Geometry check sheet. Reference: drawing and pictorial views, mm from the part's lowest x, y, z. A direction names the side the tool comes from. Coordinates: 2 decimals unless noted, no trailing zeros. Order: outer loops, then holes, each group sorted by start corner. A loop starts at its lowest first (then second) coordinate and runs counter-clockwise, first axis right, second up. Notation, with made-up numbers: M -24,41.5 L 2,41.5 A26 cw 2,63.5 Z; hole C -10,-28 d1. An arc over 180 degrees is marked long. Return JSON: item names as keys, results as strings.
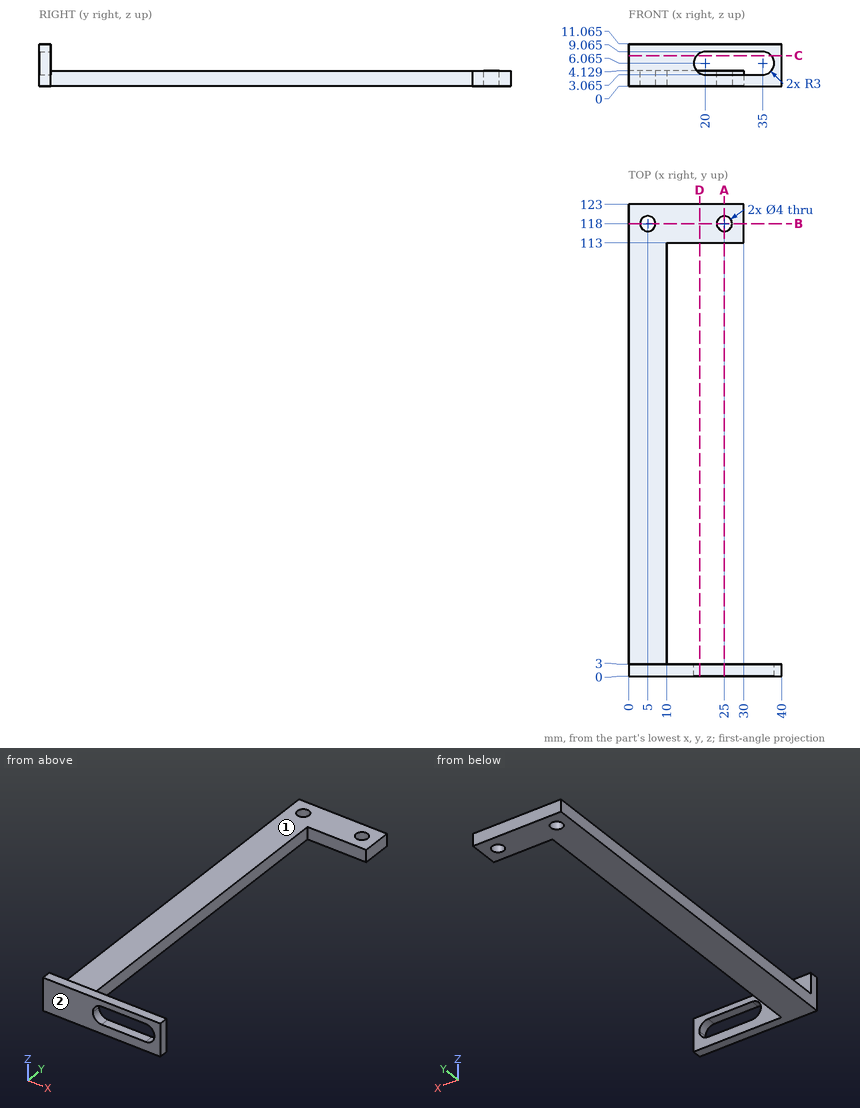
Q1. Tool access check on the marked faces 1 and 2. Record the directions out of +Z, -Z, +X, -X, +Y, -Y that give a thin tool (end or side, any length) a straight path to the whole face; none if there is none.
Values:
{"face 1": "+Z, +X, -X, +Y", "face 2": "+Z, -Z, +X, -X, -Y"}
Q2. Cross-section at B-B, the plane y = 118. Record the boundary of the cut face in (x, z).
Values:
{"outline": "M 0,0 L 3,0 L 3,4.13 L 0,4.13 Z; M 7,0 L 23,0 L 23,4.13 L 7,4.13 Z; M 27,0 L 30,0 L 30,4.13 L 27,4.13 Z"}
Q3. Cross-section at A-A, the plane x = 25. Record the boundary of the cut face in (y, z) (1 decimal).
Values:
{"outline": "M 0,0 L 3,0 L 3,3.1 L 0,3.1 Z; M 0,9.1 L 3,9.1 L 3,11.1 L 0,11.1 Z; M 113,0 L 116,0 L 116,4.1 L 113,4.1 Z; M 120,0 L 123,0 L 123,4.1 L 120,4.1 Z"}
Q4. Material ranges on line 1 along Y through (x, z) = (13.5, 1); line 2 along Y through (x, z) = (5, 2.35); line 3 along Y through (x, z) = (8, 6), recorded low to high.
Values:
{"line 1": "0 to 3, 113 to 123", "line 2": "0 to 116, 120 to 123", "line 3": "0 to 3"}
Q5. Cross-section at C-C, the plane z = 8. Record the boundary of the cut face in (x, y).
Values:
{"outline": "M 0,0 L 17.71,0 L 17.71,3 L 0,3 Z; M 37.29,0 L 40,0 L 40,3 L 37.29,3 Z"}
Q6. Go/stop test with flat-tipped pins: pin 1 (10 mm diameter, centred on x = 8.5, y = 29.5, fed in from +Z); pin 2 (2 mm diameter, centred on y = 63.5, z = 2, fed in from +X); pin 3 (3.5 mm diameter, centred on y = 120, z = 2.5, fed in from +X); pin 4 (3 mm diameter, centred on x = 25, y = 118, fed in from -Z). Record where each tip stops, or that it passes through.
Values:
{"pin 1": "z = 4.13", "pin 2": "x = 10", "pin 3": "x = 30", "pin 4": "through"}
Q7. Cross-section at D-D, the plane x = 18.5. Record the boundary of the cut face in (y, z) (1 decimal), and give its area (3 significant figures).
Values:
{"outline": "M 0,0 L 3,0 L 3,3.5 L 0,3.5 Z; M 0,8.7 L 3,8.7 L 3,11.1 L 0,11.1 Z; M 113,0 L 123,0 L 123,4.1 L 113,4.1 Z", "area": "58.9 mm^2"}
